from build123d import *

# Parameters (mm, degrees)
F0_R     = 10.5
F0_R_2   = 5
F1_DEPTH = 1.75
F0_R_3   = 4.1
F2_DEPTH = 6
F3_DEPTH = 2.5
F5_R     = 1


with BuildPart() as f1:
    # F0 (on Top) → F1 (new body)
    with BuildSketch(Plane.XY):
        Circle(F0_R)
        Circle(F0_R_2, mode=Mode.SUBTRACT)
    extrude(amount=F1_DEPTH)


with BuildPart() as f2:
    # F0 (on Top) → F2 (new body)
    with BuildSketch(Plane.XY):
        Circle(F0_R_3)
    extrude(amount=F2_DEPTH)


with BuildPart() as f3:
    # F0 (on Top) → F3 (new body)
    with BuildSketch(Plane.XY):
        Circle(F0_R_2)
        Circle(F0_R_3, mode=Mode.SUBTRACT)
    extrude(amount=F3_DEPTH)


with BuildPart() as f1_1:
    add(f1.part)

    # F4: union F3, F2
    add(f3.part)
    add(f2.part)

    # F5
    f5_edges = [f1_1.edges().sort_by_distance(p)[0] for p in [
        (-10.5, 0, 0),
    ]]
    fillet(f5_edges, radius=F5_R)


solid = f1_1.part
Verification items for the finished model (mm, model axes). A direction names the side the tool comes from. Coordinates: 2 decimals unless noted, no trailing zeros. Write each loop counter-clockwise with the first axis right and the second up, starting at its lowest first coordinate (ties: lowest second). Pieces come first, ordered by that corner, then holes. Notation, with made-up numbers: M 60.5,33.5 L 86.5,33.5 A25 cw 86.5,55.5 Z; hole C -33,36 d4. An arc over 180 degrees is marked long. Use a Markdown table: item, result.
Q1. Sectioned sample at C-C, the plane z = 5.25. Record the boundary of the cut face in (x, y).
Reply:
| item | result |
|---|---|
| outline | C 0,0 d8.2 |
Q2. Sectioned sample at B-B, the plane z = 1.25. Record the boundary of the cut face in (x, y).
Reply:
| item | result |
|---|---|
| outline | C 0,0 d21 |
Q3. Set-up check for faces 1 (the face through (0, 0, 6)), 2 (the face through (-4, 2, 2.5)): record each of +Z, -Z, +X, -X, +Y, -Y from which the full face is reachable in a straight line by a thin tool's end or side.
Reply:
| item | result |
|---|---|
| face 1 | +Z, +X, -X, +Y, -Y |
| face 2 | +Z |
Q4. Thickness scan on line 1 (Z direction, x = -2, y = 7.75); line 2 (Z direction, x = 3.75, y = -2.25); line 3 (X direction, y = 0.25, z = 1). Record the ranges inside material, lowest first.
Reply:
| item | result |
|---|---|
| line 1 | z = 0 to 1.75 |
| line 2 | z = 0 to 2.5 |
| line 3 | x = -10.5 to 10.5 |
Q5. Go/stop test with flat-tipped pins: P1, Ø1, axis at x = -2, y = 1, coming from the -Z side; P2, Ø2, axis at x = 5, z = 1.5, coming from the +Y side; P3, Ø2, axis at x = -4.5, y = -3, coming from the +Z side. Record where each tip stops, or that it passes through.
Reply:
| item | result |
|---|---|
| P1 | stops at z = 0 |
| P2 | stops at y = 9.71 |
| P3 | stops at z = 2.5 |
Q6. Sectioned sample at A-A, the plane x = 0. Record the boundary of the cut face in (y, z), plus the area to 3 significant figures.
Reply:
| item | result |
|---|---|
| outline | M -10.5,1 A1 ccw -9.5,0 L 9.5,0 A1 ccw 10.5,1 L 10.5,1.75 L 5,1.75 L 5,2.5 L 4.1,2.5 L 4.1,6 L -4.1,6 L -4.1,2.5 L -5,2.5 L -5,1.75 L -10.5,1.75 Z |
| area | 72.5 mm² |
